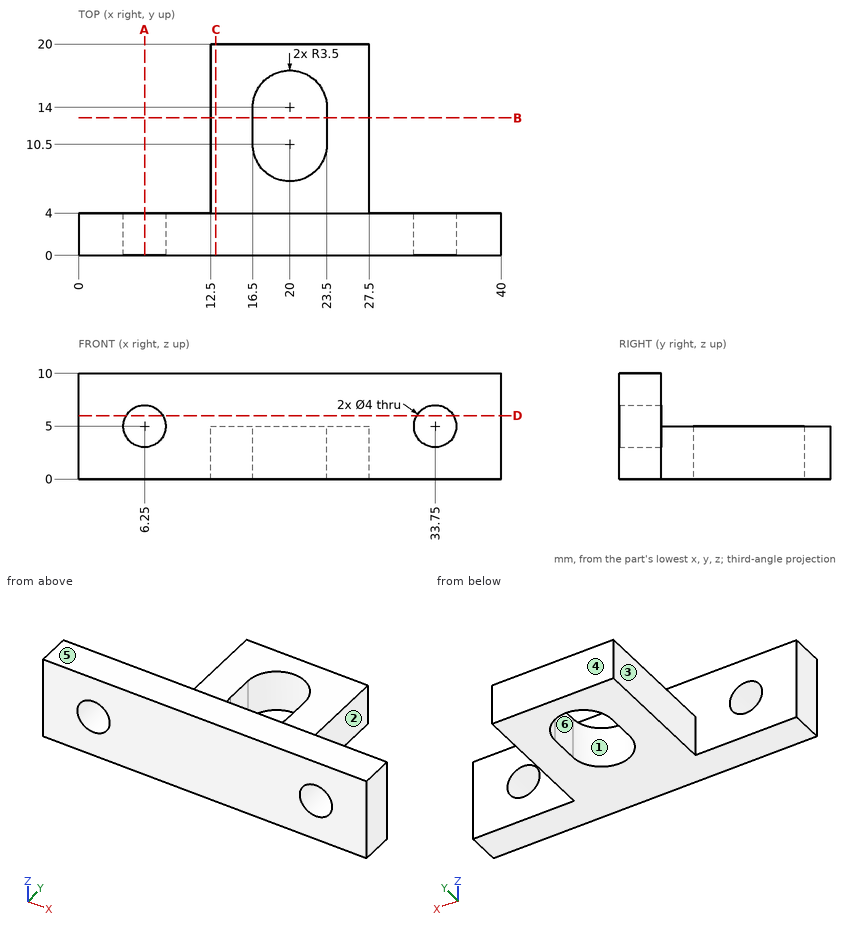
Can you work these out from the drawing? Everything is in mm from the part's minimum corner. A direction names the side the tool comes from. Coordinates: 2 decimals unless noted, no trailing zeros. Order: outer loops, then holes, each group sorted by start corner. A loop starts at its lowest first (then second) coordinate and runs counter-clockwise, first axis right, second up. Notation, with made-up numbers: M -31.75,9.5 L -8.75,9.5 A31 ccw -8.75,44.5 Z; hole C 33,78 d3. An arc over 180 degrees is marked long. Answer as CSV lines item,"result". Start each with the question number.
1. I want a section at D-D, the plane z = 6. Write out the boundary of the cut face in (x, y), and give its area (3 significant figures).
2. I want a section at C-C, the plane x = 13. Write out the boundary of the cut face in (y, z).
3. We'd pull the mould along Y, two halves only. Please class the marked faces 4, 5 and 6: released by +Y, released by -Y, zero draft, split by the parting line, or undercut.
4. I need wall thicknesses on line 1 (X direction, y = 2.4, z = 5); line 2 (Z direction, x = 6.25, y = 3); line 3 (Z direction, x = 25, y = 8). Which ranges of each line are inside material? Lowest first, please. Write a range as [from, to].
5. On a 3-axis mill with a long thin cutter (end or side, diameter ignored), from which of +Z, -Z, +X, -X, +Y, -Y can I reach the whole of each face in a straight line? I mean the marked faces 1, 2 and 3. Say none if no direction works.
6. I want a section at A-A, the plane x = 6.25. Write out the boundary of the cut face in (y, z).
7. I want a section at B-B, the plane y = 13. Write out the boundary of the cut face in (x, z).
8. For pin 1 (12 mm diameter, centred on x = 22.5, y = 11.5, fed in from +Z); pin 2 (1 mm diameter, centred on y = 11.5, z = 3, fed in from -X); pin 3 (1.5 mm diameter, centred on y = 9, z = 1.5, fed in from +X), each with a flat end and sliding along its axis, tell me the tip position at first contact or that it passes through.
Recorded:
1,outline,"M 0,0 L 4.52,0 L 4.52,4 L 0,4 Z; M 7.98,0 L 32.02,0 L 32.02,4 L 7.98,4 Z; M 35.48,0 L 40,0 L 40,4 L 35.48,4 Z"
1,area,"132 mm2"
2,outline,"M 0,0 L 20,0 L 20,5 L 4,5 L 4,10 L 0,10 Z"
3,face 4,"released by +Y"
3,face 5,"zero draft"
3,face 6,"undercut"
4,line 1,"x = [0, 4.25], [8.25, 31.75], [35.75, 40]"
4,line 2,"z = [0, 3], [7, 10]"
4,line 3,"z = [0, 5]"
5,face 1,"+Z, -Z"
5,face 2,"+Z, -Z, +X, +Y"
5,face 3,"+Z, -Z, -X, +Y"
6,outline,"M 0,0 L 4,0 L 4,3 L 0,3 Z; M 0,7 L 4,7 L 4,10 L 0,10 Z"
7,outline,"M 12.5,0 L 16.5,0 L 16.5,5 L 12.5,5 Z; M 23.5,0 L 27.5,0 L 27.5,5 L 23.5,5 Z"
8,pin 1,"stops at z = 5"
8,pin 2,"stops at x = 12.5"
8,pin 3,"stops at x = 27.5"
